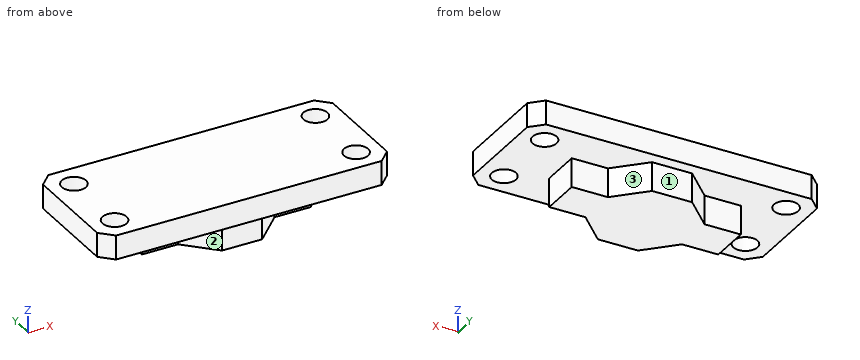
from build123d import *

# Parameters (mm, degrees)
SKETCH_156_W          = 120
SKETCH_156_H          = 50
EXTRUDE_416_DEPTH     = 10
CUT_EXTRUDE_START     = 10
SKETCH_1_5_R          = 5
CUT_EXTRUDE_465_DEPTH = 10
CHAMFER_532_SIZE      = 5
EXTRUDE_START         = -10
EXTRUDE_2_DEPTH       = 22


with BuildPart() as part:
    # Sketch 156 → Extrude 416 (new body)
    with BuildSketch(Plane.XY):
        Rectangle(SKETCH_156_W, SKETCH_156_H)
    extrude(amount=EXTRUDE_416_DEPTH)

    # Эскиз1<5> → Cut-Extrude 465 (cut)
    with BuildSketch(Plane.XY.offset(CUT_EXTRUDE_START)):
        with Locations((50, 15)):
            Circle(SKETCH_1_5_R)
        with Locations(Location((-50, 15, 0), (0, 0, 180))):
            Circle(SKETCH_1_5_R)
        with Locations((-50, -15)):
            Circle(SKETCH_1_5_R)
        with Locations(Location((50, -15, 0), (0, 0, 180))):
            Circle(SKETCH_1_5_R)
    extrude(amount=-CUT_EXTRUDE_465_DEPTH, mode=Mode.SUBTRACT)

    # Chamfer 532
    chamfer_532_edges = [part.edges().sort_by_distance(p)[0] for p in [
        (-60, 25, 5),
        (60, 25, 5),
        (60, -25, 5),
        (-60, -25, 5),
    ]]
    chamfer(chamfer_532_edges, length=CHAMFER_532_SIZE)

    # Эскиз2 → Бобышка-Вытянуть2 (add)
    with BuildSketch(Plane(origin=(0, 0, 0), x_dir=(-1, 0, 0), z_dir=(0, 0, -1)).offset(EXTRUDE_START)):
        Polygon((-8.3, 20), (8.3, 20), (20, 8.3), (35, 8.3), (35, -8.3), (20, -8.3), (8.3, -20), (-8.3, -20), (-20, -8.3), (-35, -8.3), (-35, 8.3), (-20, 8.3), align=None)
    extrude(amount=EXTRUDE_2_DEPTH)


solid = part.part
Input: part model. Units: mm. Frame: model coordinates. Face numbers are marked on the shaded views. A direction names the side the tool comes from. Coordinates: 2 decimals unless noted, no trailing zeros. Loops run counter-clockwise (first coordinate to the right, second up) from the corner with the lowest first, then second, coordinate; pieces in that order, holes last. Notation, with made-up numbers: (9.5, 55) - (54.5, 55) arc R21 cw to (54.5, 86) - close; hole circle Ø10 at (-29.5, 75). An arc over 180 degrees is marked (long way). Answer in a Markdown table with one row per item. Add a question column.
Item 1: Section query B-B on y = -12. Return the cut outline in (x, z).
Item 2: Section query C-C on z = 2.75. Return the cut outline in (x, y).
Item 3: Line query: line 1 along Y through (x, z) = (50, 5.75); line 2 along Y through (x, z) = (-48, 1); line 3 along X through (y, z) = (11.5, 3.25). Output: solid intervals per line, ascending. Write a range as [from, to].
Item 4: Contact query for flat-ended pins moving along their axis: P1, Ø3.5, axis at x = -24.5, z = -7.5, coming from the -Y side; P2, Ø1, axis at y = -1.5, z = -2, coming from the -X side; P3, Ø8, axis at x = 47.5, z = -7, coming from the -Y side; P4, Ø11.5, axis at x = -50, y = -15, coming from the -Z side. Output: stop coordinate, or through.
Item 5: Section query A-A on x = 50. Return the cut outline in (y, z).
Item 6: Section query D-D on y = 5. Return the cut outline in (x, z), then the cut area to 3 significant figures.
Item 7: Access query for the marked faces 1, 2 and 3. Directions: +Z, -Z, +X, -X, +Y, -Y. A direction counts if a zero-diameter tool reaches every point of the face in a straight line with its end or side. Return the directions, or none.
Recorded:
| question | item | result |
|---|---|---|
| 1 | outline | (-60, 0) - (-54, 0) - (-54, 10) - (-60, 10) - close; (-46, 0) - (-16.3, 0) - (-16.3, -12) - (16.3, -12) - (16.3, 0) - (46, 0) - (46, 10) - (-46, 10) - close; (54, 0) - (60, 0) - (60, 10) - (54, 10) - close |
| 2 | outline | (-60, -20) - (-55, -25) - (55, -25) - (60, -20) - (60, 20) - (55, 25) - (-55, 25) - (-60, 20) - close; hole circle Ø10 at (-50, -15); hole circle Ø10 at (-50, 15); hole circle Ø10 at (50, -15); hole circle Ø10 at (50, 15) |
| 3 | line 1 | [-25, -20], [-10, 10], [20, 25] |
| 3 | line 2 | [-25, -19.58], [-10.42, 10.42], [19.58, 25] |
| 3 | line 3 | [-60, -53.57], [-46.43, 46.43], [53.57, 60] |
| 4 | P1 | y = -8.3 |
| 4 | P2 | x = -35 |
| 4 | P3 | through |
| 4 | P4 | z = 0 |
| 5 | outline | (-25, 0) - (-20, 0) - (-20, 10) - (-25, 10) - close; (-10, 0) - (10, 0) - (10, 10) - (-10, 10) - close; (20, 0) - (25, 0) - (25, 10) - (20, 10) - close |
| 6 | outline | (-60, 0) - (-35, 0) - (-35, -12) - (35, -12) - (35, 0) - (60, 0) - (60, 10) - (-60, 10) - close |
| 6 | area | 2,040 mm^2 |
| 7 | face 1 | -Z, +X, -X, +Y |
| 7 | face 2 | -Z, -X, -Y |
| 7 | face 3 | -Z, +X, +Y |
